For this review, take the finished solid that the model builds, in its own axes (mm). A direction names the side the tool comes from. Give positions to 0.01 mm unless a question says otherwise; leave off trailing zeros. Loops run counter-clockwise (first coordinate to the right, second up) from the corner with the lowest first, then second, coordinate; pieces in that order, holes last.
```python
from build123d import *

# Parameters (mm, degrees)
SKETCH1_W                                    = 50
SKETCH1_H                                    = 50
BOSS_EXTRUDE1_DEPTH                          = 3
SKETCH3_W                                    = 50
SKETCH3_H                                    = 50
SKETCH3_W_2                                  = 42.5
SKETCH3_H_2                                  = 42.5
BOSS_EXTRUDE2_DEPTH                          = 39.7
CUT_EXTRUDE5_START                           = -5
SKETCH19_W                                   = 16.15
SKETCH19_H                                   = 9.6
CUT_EXTRUDE5_DEPTH                           = 76.344082907
SKETCH33_W                                   = 25
SKETCH33_H                                   = 5.25
BOSS_EXTRUDE14_DEPTH                         = 5
SKETCH21_R                                   = 1.7
CUT_EXTRUDE6_DEPTH                           = 5
CUT_EXTRUDE8_REACH                           = 59.864
SKETCH27_R                                   = 11.5
CSK_FOR_M3_COUNTERSUNK_FLAT_HEAD_SCR_2_COUNT = 2
CSK_FOR_M3_COUNTERSUNK_FLAT_HEAD_SCR_2_PITCH = 31
CSK_FOR_M3_COUNTERSUNK_FLAT_HEAD_SCR_3_COUNT = 2
CSK_FOR_M3_COUNTERSUNK_FLAT_HEAD_SCR_3_PITCH = 43.840620434
CSK_FOR_M3_COUNTERSUNK_FLAT_HEAD_SCR_4_COUNT = 2
CSK_FOR_M3_COUNTERSUNK_FLAT_HEAD_SCR_4_PITCH = 31
SKETCH34_W                                   = 17.78
SKETCH34_H                                   = 10.2616
BOSS_EXTRUDE15_DEPTH                         = 4.9784
SKETCH35_W                                   = 17.78
SKETCH35_H                                   = 2.4384
BOSS_EXTRUDE16_DEPTH                         = 4.9784
CIRPATTERN1_COUNT                            = 4
CIRPATTERN1_COPY_1_SKETCH_W                  = 17.78
CIRPATTERN1_COPY_1_SKETCH_H                  = 2.4384
CIRPATTERN1_COPY_1_DEPTH                     = 4.9784
CIRPATTERN1_COPY_2_SKETCH_W                  = 17.78
CIRPATTERN1_COPY_2_SKETCH_H                  = 2.4384
CIRPATTERN1_COPY_2_DEPTH                     = 4.9784
CIRPATTERN1_COPY_3_SKETCH_W                  = 17.78
CIRPATTERN1_COPY_3_SKETCH_H                  = 2.4384
CIRPATTERN1_COPY_3_DEPTH                     = 4.9784


with BuildPart() as part:
    # Sketch1 → Boss-Extrude1 (new body)
    with BuildSketch(Plane(origin=(0, 0, 0), x_dir=(1, 0, 0), z_dir=(0, 1, 0))):
        Rectangle(SKETCH1_W, SKETCH1_H)
    extrude(amount=BOSS_EXTRUDE1_DEPTH)

    # Sketch3 → Boss-Extrude2 (add)
    with BuildSketch(Plane(origin=(0, 3, 0), x_dir=(1, 0, 0), z_dir=(0, 1, 0))):
        Rectangle(SKETCH3_W, SKETCH3_H)
        Rectangle(SKETCH3_W_2, SKETCH3_H_2, mode=Mode.SUBTRACT)
    extrude(amount=BOSS_EXTRUDE2_DEPTH)

    # Sketch19 → Cut-Extrude5 (cut)
    with BuildSketch(Plane(origin=(25, 0, 0), x_dir=(0, 0, -1), z_dir=(1, 0, 0)).offset(CUT_EXTRUDE5_START)):
        with Locations((0, 37.9)):
            Rectangle(SKETCH19_W, SKETCH19_H)
    cut_extrude5 = extrude(amount=CUT_EXTRUDE5_DEPTH, mode=Mode.SUBTRACT)

    # Sketch33 → Boss-Extrude14 (add)
    with BuildSketch(Plane.XY.offset(25)):
        with Locations((0, 40.075)):
            Rectangle(SKETCH33_W, SKETCH33_H)
    boss_extrude14 = extrude(amount=BOSS_EXTRUDE14_DEPTH)

    # Mirror7: Boss-Extrude14 across plane
    add(boss_extrude14.mirror(Plane.XY))

    # Sketch21 → Cut-Extrude6 (cut)
    with BuildSketch(Plane(origin=(0, 42.7, 0), x_dir=(1, 0, 0), z_dir=(0, 1, 0))):
        with Locations(Location((5, -25.25, 0), (0, 0, 270))):
            Circle(SKETCH21_R)
        with Locations(Location((-5, 25.25, 0), (0, 0, 270))):
            Circle(SKETCH21_R)
        with Locations(Location((5, 25.25, 0), (0, 0, 270))):
            Circle(SKETCH21_R)
        with Locations(Location((-5, -25.25, 0), (0, 0, 270))):
            Circle(SKETCH21_R)
    extrude(amount=-CUT_EXTRUDE6_DEPTH, mode=Mode.SUBTRACT)

    # Sketch27 → Cut-Extrude8 (cut, up to next)
    with BuildSketch(Plane.XZ, mode=Mode.PRIVATE) as cut_extrude8_sk1:
        with Locations(Location((0, 0, 0), (0, 0, 270))):
            Circle(SKETCH27_R)
    cut_extrude8_tool1 = extrude(cut_extrude8_sk1.sketch, amount=-CUT_EXTRUDE8_REACH, mode=Mode.PRIVATE) & part.part
    add(cut_extrude8_tool1.solids().sort_by_distance((0, 0, 0))[0], mode=Mode.SUBTRACT)

    # Sketch30 → CSK for M3 Countersunk Flat Head Screw1 (revolve, cut)
    with BuildSketch(Plane(origin=(-15.5, 0, 15.5), x_dir=(0, 0, -1), z_dir=(1, 0, 0))):
        Polygon((0, 0), (0, 3), (1.7, 3), (1.7, 1.45), (3.15, 0), align=None)
    csk_for_m3_countersunk_flat_head_screw1 = revolve(axis=Axis((-15.5, -6.35, 15.5), (0, 1, 0)), mode=Mode.SUBTRACT)

    # CSK for M3 Countersunk Flat Head Scr 2: CSK for M3 Countersunk Flat Head Screw1 ×2
    with Locations(*[(i * CSK_FOR_M3_COUNTERSUNK_FLAT_HEAD_SCR_2_PITCH, 0, 0) for i in range(1, CSK_FOR_M3_COUNTERSUNK_FLAT_HEAD_SCR_2_COUNT)]):
        add(csk_for_m3_countersunk_flat_head_screw1, mode=Mode.SUBTRACT)

    # CSK for M3 Countersunk Flat Head Scr 3: CSK for M3 Countersunk Flat Head Screw1 ×2
    with Locations(*[Vector(0.7071067811865475, 0, -0.7071067811865476) * (i * CSK_FOR_M3_COUNTERSUNK_FLAT_HEAD_SCR_3_PITCH) for i in range(1, CSK_FOR_M3_COUNTERSUNK_FLAT_HEAD_SCR_3_COUNT)]):
        add(csk_for_m3_countersunk_flat_head_screw1, mode=Mode.SUBTRACT)

    # CSK for M3 Countersunk Flat Head Scr 4: CSK for M3 Countersunk Flat Head Screw1 ×2
    with Locations(*[(0, 0, -i * CSK_FOR_M3_COUNTERSUNK_FLAT_HEAD_SCR_4_PITCH) for i in range(1, CSK_FOR_M3_COUNTERSUNK_FLAT_HEAD_SCR_4_COUNT)]):
        add(csk_for_m3_countersunk_flat_head_screw1, mode=Mode.SUBTRACT)

    # Mirror4: Cut-Extrude5 across plane
    add(cut_extrude5.mirror(Plane(origin=(0, 0, 0), x_dir=(0, 0, 1), z_dir=(1, 0, 0))), mode=Mode.SUBTRACT)

    # Sketch34 → Boss-Extrude15 (add)
    with BuildSketch(Plane.XY.offset(25)):
        with Locations((0, 15.3416)):
            Rectangle(SKETCH34_W, SKETCH34_H)
    boss_extrude15 = extrude(amount=BOSS_EXTRUDE15_DEPTH)

    # Sketch35 → Boss-Extrude16 (add)
    with BuildSketch(Plane(origin=(0, 20.4724, 0), x_dir=(1, 0, 0), z_dir=(0, 1, 0))):
        with Locations((0, -28.7592)):
            Rectangle(SKETCH35_W, SKETCH35_H)
    boss_extrude16 = extrude(amount=BOSS_EXTRUDE16_DEPTH)

    # Mirror8: Boss-Extrude16 across plane
    add(boss_extrude16.mirror(Plane.ZX.offset(15.3416)))

    # CirPattern1: Boss-Extrude15, Boss-Extrude16 ×4 about axis
    cirpattern1_axis = Axis((0, 0, 0), (0, 1, 0))
    add([boss_extrude15.rotate(cirpattern1_axis, i * 360 / CIRPATTERN1_COUNT) for i in range(1, CIRPATTERN1_COUNT)])
    add([boss_extrude16.rotate(cirpattern1_axis, i * 360 / CIRPATTERN1_COUNT) for i in range(1, CIRPATTERN1_COUNT)])

    # CirPattern1 copy 1 sketch → CirPattern1 copy 1 (add)
    with BuildSketch(Plane(origin=(0, 10.2108, 0), x_dir=(0, 0, -1), z_dir=(0, -1, 0))):
        with Locations((0, 28.7592)):
            Rectangle(CIRPATTERN1_COPY_1_SKETCH_W, CIRPATTERN1_COPY_1_SKETCH_H)
    extrude(amount=CIRPATTERN1_COPY_1_DEPTH)

    # CirPattern1 copy 2 sketch → CirPattern1 copy 2 (add)
    with BuildSketch(Plane(origin=(0, 10.2108, 0), x_dir=(-1, 0, 0), z_dir=(0, -1, 0))):
        with Locations((0, 28.7592)):
            Rectangle(CIRPATTERN1_COPY_2_SKETCH_W, CIRPATTERN1_COPY_2_SKETCH_H)
    extrude(amount=CIRPATTERN1_COPY_2_DEPTH)

    # CirPattern1 copy 3 sketch → CirPattern1 copy 3 (add)
    with BuildSketch(Plane(origin=(0, 10.2108, 0), x_dir=(0, 0, 1), z_dir=(0, -1, 0))):
        with Locations((0, 28.7592)):
            Rectangle(CIRPATTERN1_COPY_3_SKETCH_W, CIRPATTERN1_COPY_3_SKETCH_H)
    extrude(amount=CIRPATTERN1_COPY_3_DEPTH)


solid = part.part
```
Item 1: Tool access review of faces 1 (the flat face through (29, 25.451, 0)), 2 (the flat face through (-23, 33.1, 0)), 3 (the cylindrical face through (4.3, 40.2, 26.8)), 4 (the flat face through (0, 25.451, -29)): name each direction out of +Z, -Z, +X, -X, +Y, -Y from which nothing blocks a thin tool from reaching the whole face with its end or side.
Answer:
face 1: +Z, -Z, +X, +Y
face 2: +X, -X, +Y
face 3: +Y
face 4: -Z, +X, -X
Item 2: The part is to be moulded in two halves that separate along Y. For faces 5 (the flat face through (0, 23, 27.54)), 6 (the flat face through (-27.54, 8, 0)), 7 (the flat face through (0, 25.451, 29)), 8 (the flat face through (5, 37.7, 25)), say which applies: released by +Y, released by -Y, zero draft, split by the parting line, or undercut.
Answer:
face 5: undercut
face 6: zero draft
face 7: undercut
face 8: released by +Y
Item 3: Take a section at D-D on z = 0. Give the boundary of the cut face in (x, y), and give its area (3 significant figures).
Answer:
outline: (-29.98, 5.23) - (-27.54, 5.23) - (-27.54, 10.21) - (-25, 10.21) - (-25, 0) - (-11.5, 0) - (-11.5, 3) - (-21.25, 3) - (-21.25, 33.1) - (-25, 33.1) - (-25, 20.47) - (-27.54, 20.47) - (-27.54, 25.45) - (-29.98, 25.45) - close; (11.5, 0) - (25, 0) - (25, 10.21) - (27.54, 10.21) - (27.54, 5.23) - (29.98, 5.23) - (29.98, 25.45) - (27.54, 25.45) - (27.54, 20.47) - (25, 20.47) - (25, 33.1) - (21.25, 33.1) - (21.25, 3) - (11.5, 3) - close
area: 457 mm2
Item 4: Take a section at A-A on y = 8.5. Give the boundary of the cut face in (x, z).
Answer:
outline: (-29.98, -8.89) - (-27.54, -8.89) - (-27.54, 8.89) - (-29.98, 8.89) - close; (-25, -25) - (25, -25) - (25, 25) - (-25, 25) - close; (-8.89, -29.98) - (8.89, -29.98) - (8.89, -27.54) - (-8.89, -27.54) - close; (-8.89, 27.54) - (8.89, 27.54) - (8.89, 29.98) - (-8.89, 29.98) - close; (27.54, -8.89) - (29.98, -8.89) - (29.98, 8.89) - (27.54, 8.89) - close; hole (-21.25, -21.25) - (21.25, -21.25) - (21.25, 21.25) - (-21.25, 21.25) - close
Item 5: Take a section at C-C on z = -15.5. Give the boundary of the cut face in (x, y).
Answer:
outline: (-25, 0) - (-18.65, 0) - (-17.2, 1.45) - (-17.2, 3) - (-21.25, 3) - (-21.25, 42.7) - (-25, 42.7) - close; (-13.8, 1.45) - (-12.35, 0) - (12.35, 0) - (13.8, 1.45) - (13.8, 3) - (-13.8, 3) - close; (17.2, 1.45) - (18.65, 0) - (25, 0) - (25, 42.7) - (21.25, 42.7) - (21.25, 3) - (17.2, 3) - close
Item 6: For L1, parallel to X at y = 24, z = 7; L2, parallel to Z at x = -15.5, y = 2.5; L3, parallel to X at y = 14, z = -1, list the stretches that pass through material, from the lowest coordinate up.
Answer:
L1: x = -29.98 to -27.54, -25 to -21.25, 21.25 to 25, 27.54 to 29.98
L2: z = -25 to -17.2, -13.8 to 13.8, 17.2 to 25
L3: x = -29.98 to -21.25, 21.25 to 29.98
Item 7: Clearance check with flat-ended pins moving along their axes: pin 1 Ø3 at (x, y) = (16, 15) entering from +Z; pin 2 Ø13 at (x, y) = (-11, 14.5) entering from +Z; pin 3 Ø4 at (y, z) = (39.5, -27.5) entering from +X; pin 4 Ø3 at (x, z) = (15.5, 15.5) entering from -Y. State where each tip first meets the part, or that it passes through.
Answer:
pin 1: stops at z = 25
pin 2: stops at z = 29.98
pin 3: stops at x = 12.5
pin 4: passes through
